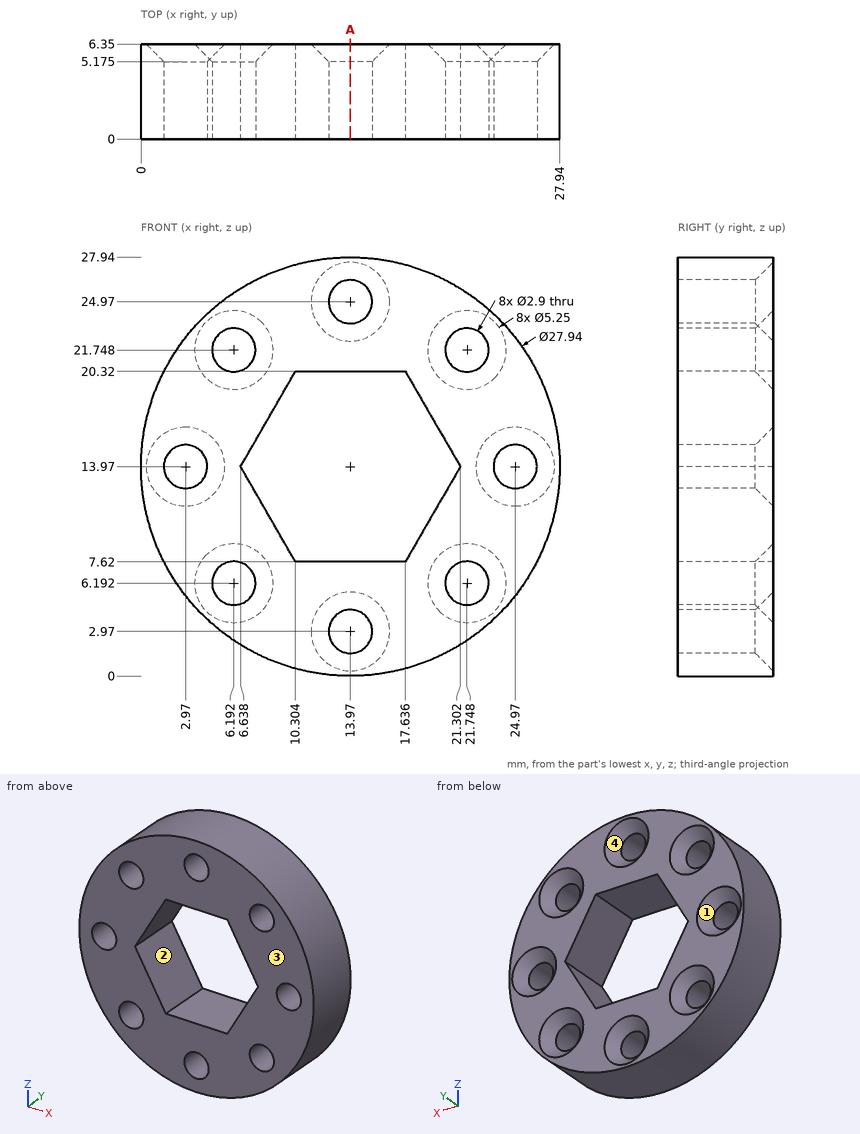
Job drawing, mm, ordinate dimensions from the low corner. One solid piece. A direction names the side the tool comes from. Round coordinates to 2 decimals unless told otherwise and drop trailing zeros. One line per question, with ' | ' between items. Start each with the question number.
Item 1: Which spindle directions (+Z, -Z, +X, -X, +Y, -Y) get a long thin tool onto all of the face, cutting with end or side? Do the marked faces 1 and 2. Say none if no direction does.
Item 2: Wall check: line 1 (X direction, y = 3.5, z = 22.5) (1 decimal); line 2 (Z direction, x = 15.25, y = 5.25); line 3 (X direction, y = 3.25, z = 14.25). Give the ranges that are in metal, low to high.
Item 3: Pin check, flat tips, straight feed: pin 1 Ø2 at (x, y) = (12, 3) entering from +Z; pin 2 Ø4.5 at (x, z) = (2.97, 13.97) entering from +Y (1 decimal). Stop position of each tip, or through.
Item 4: Cut at A-A, the plane x = 13.97. State how many separate pieces and enclosed holes the cut face has.
Item 5: Two-plate mould, pull along Z, no slides. Class the marked faces 3 and 4: pulls with the +Z half, pulls with the -Z half, needs draft (parallel to the pull), parting line crosses it, or undercut.
Responses:
1) face 1: +Y | face 2: +Y, -Y
2) line 1: x = 2.9 to 5, 7.4 to 20.5, 23 to 25 | line 2: z = 0.06 to 2.14, 3.8 to 7.62, 20.32 to 24.14, 25.8 to 27.88 | line 3: x = 0 to 1.55, 4.39 to 6.8, 21.14 to 23.55, 26.39 to 27.94
3) pin 1: stops at z = 27.91 | pin 2: stops at y = 6
4) separate pieces: 4 | enclosed holes: 0
5) face 3: needs draft | face 4: undercut
